```python
from build123d import *

# Parameters (mm, degrees)
SKETCH1_R           = 17.375
BOSS_EXTRUDE1_DEPTH = 2.04
SKETCH2_R           = 14.3
BOSS_EXTRUDE2_DEPTH = 4.83
SKETCH3_R           = 2.74
BOSS_EXTRUDE3_DEPTH = 40.36
SKETCH4_R           = 17.375
BOSS_EXTRUDE4_DEPTH = 2.04
SKETCH5_R           = 14.3
BOSS_EXTRUDE5_DEPTH = 4.83
SKETCH6_R           = 1.485
BOSS_EXTRUDE6_DEPTH = 8.5
SKETCH7_R           = 1.485
BOSS_EXTRUDE7_DEPTH = 8.5


with BuildPart() as part:
    # Sketch1 → Boss-Extrude1 (new body)
    with BuildSketch(Plane.XY):
        Circle(SKETCH1_R)
    extrude(amount=BOSS_EXTRUDE1_DEPTH)

    # Sketch2 → Boss-Extrude2 (add)
    with BuildSketch(Plane.XY.offset(2.04)):
        Circle(SKETCH2_R)
    extrude(amount=BOSS_EXTRUDE2_DEPTH)

    # Sketch3 → Boss-Extrude3 (add)
    with BuildSketch(Plane(origin=(0, 0, 0), x_dir=(-1, 0, 0), z_dir=(0, 0, -1))):
        Circle(SKETCH3_R)
    extrude(amount=BOSS_EXTRUDE3_DEPTH)

    # Sketch4 → Boss-Extrude4 (add)
    with BuildSketch(Plane(origin=(0, 0, -40.36), x_dir=(-1, 0, 0), z_dir=(0, 0, -1))):
        Circle(SKETCH4_R)
    extrude(amount=BOSS_EXTRUDE4_DEPTH)

    # Sketch5 → Boss-Extrude5 (add)
    with BuildSketch(Plane(origin=(0, 0, -42.4), x_dir=(-1, 0, 0), z_dir=(0, 0, -1))):
        Circle(SKETCH5_R)
    extrude(amount=BOSS_EXTRUDE5_DEPTH)

    # Sketch6 → Boss-Extrude6 (add)
    with BuildSketch(Plane(origin=(0, 0, -47.23), x_dir=(-1, 0, 0), z_dir=(0, 0, -1))):
        Circle(SKETCH6_R)
    extrude(amount=BOSS_EXTRUDE6_DEPTH)

    # Sketch7 → Boss-Extrude7 (add)
    with BuildSketch(Plane.XY.offset(6.87)):
        Circle(SKETCH7_R)
    extrude(amount=BOSS_EXTRUDE7_DEPTH)


solid = part.part
```
Model file for the job. Use its own axes, mm. A direction names the side the tool comes from. Coordinates: 2 decimals unless noted, no trailing zeros. Loops run counter-clockwise (first coordinate to the right, second up) from the corner with the lowest first, then second, coordinate; pieces in that order, holes last. Notation, with made-up numbers: (73.5, 89.5) - (109.5, 89.5) arc R29 cw to (109.5, 112.5) - close; hole circle Ø6 at (8.5, 82.5). An arc over 180 degrees is marked (long way). Write item = value, one per line. Start each with the question number.
Item 1: Wall check: probe 1 along Z at (x, y) = (-11, -3.5); probe 2 along Z at (x, y) = (15, -3); probe 3 along Z at (x, y) = (2, -0.5). Give the ranges that are in metal, low to high. Write a range as [from, to].
Item 2: Drop flat-ended pins along their axis: pin 1 Ø12 at (x, z) = (2, -9.5) entering from -Y; pin 2 Ø2 at (x, z) = (10.5, 2.5) entering from +Y; pin 3 Ø4 at (y, z) = (1.5, -24) entering from +X. Give the stop position or say it passes through.
Item 3: Saw through at A-A, the plane x = 15. List the corners of the cut face in (y, z).
Item 4: Saw through at B-B, the plane y = 13. List the corners of the cut face in (x, z).
Item 5: Pull direction Z, two halves, no side cores. Call faces 4 (the face through (9.34, 14.65, 1.01)), 5 (the face through (-3, 0, -47.23)), 6 (the face through (4, 0, 0)), 7 (the face through (-2.613, 0.823, -19.897)): +Z half, -Z half, draft (parallel to the pull), parting line (faces both ways), or undercut.
Item 6: Saw through at C-C, the plane x = 0. List the corners of the cut face in (y, z) (3 decimals), then the cut area to 3 significant figures.
Item 7: 3-axis set-ups, long thin cutter, end or side, ignore diameter. For faces 1 (the face through (-0.32, -1.45, 11.06)), 2 (the face through (0, 0, 15.37)), 3 (the face through (14.24, -2.49, -42.4)): which of +Z, -Z, +X, -X, +Y, -Y reach the whole face in a straight line?
Answers:
q1.probe_1 = [-47.23, -40.36], [0, 6.87]
q1.probe_2 = [-42.4, -40.36], [0, 2.04]
q1.probe_3 = [-47.23, 6.87]
q2.pin_1 = -2.74
q2.pin_2 = 14.47
q2.pin_3 = 2.74
q3.outline = (-8.77, -42.4) - (8.77, -42.4) - (8.77, -40.36) - (-8.77, -40.36) - close; (-8.77, 0) - (8.77, 0) - (8.77, 2.04) - (-8.77, 2.04) - close
q4.outline = (-11.53, -42.4) - (-5.96, -42.4) - (-5.96, -47.23) - (5.96, -47.23) - (5.96, -42.4) - (11.53, -42.4) - (11.53, -40.36) - (-11.53, -40.36) - close; (-11.53, 0) - (11.53, 0) - (11.53, 2.04) - (5.96, 2.04) - (5.96, 6.87) - (-5.96, 6.87) - (-5.96, 2.04) - (-11.53, 2.04) - close
q5.face_4 = draft
q5.face_5 = -Z half
q5.face_6 = undercut
q5.face_7 = undercut
q6.outline = (-17.375, -42.4) - (-14.3, -42.4) - (-14.3, -47.23) - (-1.485, -47.23) - (-1.485, -55.73) - (1.485, -55.73) - (1.485, -47.23) - (14.3, -47.23) - (14.3, -42.4) - (17.375, -42.4) - (17.375, -40.36) - (2.74, -40.36) - (2.74, 0) - (17.375, 0) - (17.375, 2.04) - (14.3, 2.04) - (14.3, 6.87) - (1.485, 6.87) - (1.485, 15.37) - (-1.485, 15.37) - (-1.485, 6.87) - (-14.3, 6.87) - (-14.3, 2.04) - (-17.375, 2.04) - (-17.375, 0) - (-2.74, 0) - (-2.74, -40.36) - (-17.375, -40.36) - close
q6.area = 690 mm2
q7.face_1 = +Z
q7.face_2 = +Z, +X, -X, +Y, -Y
q7.face_3 = -Z
